Geometry: final body of the model. Coordinates: model frame, mm. A direction names the side the tool comes from. Round coordinates to 2 decimals unless told otherwise and drop trailing zeros. Write each loop counter-clockwise with the first axis right and the second up, starting at its lowest first coordinate (ties: lowest second). Pieces come first, ordered by that corner, then holes. Notation, with made-up numbers: M 18.25,-30.5 L 39.25,-30.5 A14 ccw 39.25,-18.5 Z; hole C 25,13 d4. An arc over 180 degrees is marked long. Use one line per item in the form item = value. Start each with the question number.
Item 1: Reachability of faces 3 (the flat face through (14.53, -6.6, 7.2)), 4 (the flat face through (-5.4, -7.08, -0.9)), 5 (the flat face through (7.4, -7.08, 7.1)), 6 (the flat face through (7, -5.31, 3)), 7 (the flat face through (-3.32, -6.6, -0.9)) from +Z, -Z, +X, -X, +Y, -Y: full face, straight path, thin tool, end or side. Return the list, or none.
Item 2: Pin query (flat end, axial travel): pin 1 Ø5 at (x, z) = (14.5, 3.5) entering from +Y; pin 2 Ø1.1 at (x, z) = (4.5, 7.5) entering from -Y; pin 3 Ø1 at (x, y) = (-2.5, -3.5) entering from -Z; pin 4 Ø0.8 at (x, z) = (15, -1.5) entering from +Y. Return the tip coordinate at first contact, or that it passes through.
Item 3: Section query C-C (x = -8.5). Return loops of the section in (y, z).
Item 4: Pull-direction query (Z, two-part tool) for faces 1 (the flat face through (-21, -1.83, 3)), 2 (the flat face through (1.78, -6.6, -0.9)); classes: pulls with the +Z half, pulls with the -Z half, needs draft (parallel to the pull), parting line crosses it, or undercut.
Item 5: Section query B-B (z = 2.5). State how many separate pieces and enclosed holes the cut face has, and give its area (3 significant figures).
Item 6: Ray query, probe 1 along Z at (x, y) = (-20.5, -5); probe 2 along Z at (x, y) = (-13.5, -1); probe 3 along Y at (x, z) = (7.5, 2.25). Return the intervals inside material, ascending.
Item 7: Section query A-A (y = -2.75). Return loops of the section in (x, z).
from build123d import *

# Parameters (mm, degrees)
SKETCH1_W             = 48.2
SKETCH1_H             = 15.7
MAIN_DEPTH            = 1.6
SKETCH2_W             = 2.54
SKETCH2_H             = 2.54
PINBASE_DEPTH         = 2.54
FILLET1_R             = 0.2
SKETCH3_W             = 1
SKETCH3_H             = 1
BOSS_EXTRUDE3_DEPTH   = 6
LPATTERN3_START       = 1.6
LPATTERN3_DEPTH       = 2.54
LPATTERN3_START_2     = -1.86
LPATTERN3_2_OUTLINE_W = 1
LPATTERN3_2_OUTLINE_H = 1
LPATTERN3_2_DEPTH     = 12
SKETCH5_W             = 8.5
SKETCH5_H             = 10.5
BOSS_EXTRUDE4_DEPTH   = 2.54
SKETCH6_W             = 1.8
SKETCH6_H             = 1.8
CUT_EXTRUDE1_DEPTH    = 6


# Read off the part's stored shape, not the designer's step: LPattern3
with BuildPart() as part:
    # Sketch1 → Main (new body)
    with BuildSketch(Plane.XY):
        Rectangle(SKETCH1_W, SKETCH1_H)
    extrude(amount=MAIN_DEPTH)

    # Sketch2 → PinBase (add)
    with BuildSketch(Plane.XY.offset(1.6)):
        with Locations((15.03, -6.58)):
            Rectangle(SKETCH2_W, SKETCH2_H)
    extrude(amount=PINBASE_DEPTH)

    # Fillet1
    fillet1_edges = [part.edges().sort_by_distance(p)[0] for p in [
        (13.76, -7.85, 2.87),
        (16.3, -7.85, 2.87),
        (16.3, -5.31, 2.87),
    ]]
    fillet(fillet1_edges, radius=FILLET1_R)

    # Sketch3 → Boss-Extrude3 (add, symmetric)
    with BuildSketch(Plane.XY.offset(4.14)):
        with Locations((15.03, -6.58)):
            Rectangle(SKETCH3_W, SKETCH3_H)
    extrude(amount=BOSS_EXTRUDE3_DEPTH, both=True)

    # LPattern3 outline → LPattern3 (add)
    with BuildSketch(Plane.XY.offset(LPATTERN3_START)):
        with BuildLine():
            Line((-6.44, -7.85), (-4.3, -7.85))
            ThreePointArc((-4.3, -7.85), (-4.158578644, -7.791421356), (-4.1, -7.65))
            Line((-4.1, -7.65), (-4.1, -5.51))
            ThreePointArc((-4.1, -5.51), (-4.158578644, -5.368578644), (-4.3, -5.31))
            Line((-4.3, -5.31), (-6.64, -5.31))
            Line((-6.64, -5.31), (-6.64, -7.65))
            ThreePointArc((-6.64, -7.65), (-6.581421356, -7.791421356), (-6.44, -7.85))
        make_face()
        with BuildLine():
            Line((-3.89, -7.85), (-1.75, -7.85))
            ThreePointArc((-1.75, -7.85), (-1.608578644, -7.791421356), (-1.55, -7.65))
            Line((-1.55, -7.65), (-1.55, -5.51))
            ThreePointArc((-1.55, -5.51), (-1.608578644, -5.368578644), (-1.75, -5.31))
            Line((-1.75, -5.31), (-4.09, -5.31))
            Line((-4.09, -5.31), (-4.09, -7.65))
            ThreePointArc((-4.09, -7.65), (-4.031421356, -7.791421356), (-3.89, -7.85))
        make_face()
        with BuildLine():
            Line((-1.34, -7.85), (0.8, -7.85))
            ThreePointArc((0.8, -7.85), (0.941421356, -7.791421356), (1, -7.65))
            Line((1, -7.65), (1, -5.51))
            ThreePointArc((1, -5.51), (0.941421356, -5.368578644), (0.8, -5.31))
            Line((0.8, -5.31), (-1.54, -5.31))
            Line((-1.54, -5.31), (-1.54, -7.65))
            ThreePointArc((-1.54, -7.65), (-1.481421356, -7.791421356), (-1.34, -7.85))
        make_face()
        with BuildLine():
            Line((1.21, -7.85), (3.35, -7.85))
            ThreePointArc((3.35, -7.85), (3.491421356, -7.791421356), (3.55, -7.65))
            Line((3.55, -7.65), (3.55, -5.51))
            ThreePointArc((3.55, -5.51), (3.491421356, -5.368578644), (3.35, -5.31))
            Line((3.35, -5.31), (1.01, -5.31))
            Line((1.01, -5.31), (1.01, -7.65))
            ThreePointArc((1.01, -7.65), (1.068578644, -7.791421356), (1.21, -7.85))
        make_face()
        with BuildLine():
            Line((3.76, -7.85), (5.9, -7.85))
            ThreePointArc((5.9, -7.85), (6.041421356, -7.791421356), (6.1, -7.65))
            Line((6.1, -7.65), (6.1, -5.51))
            ThreePointArc((6.1, -5.51), (6.041421356, -5.368578644), (5.9, -5.31))
            Line((5.9, -5.31), (3.56, -5.31))
            Line((3.56, -5.31), (3.56, -7.65))
            ThreePointArc((3.56, -7.65), (3.618578644, -7.791421356), (3.76, -7.85))
        make_face()
        with BuildLine():
            Line((6.31, -7.85), (8.45, -7.85))
            ThreePointArc((8.45, -7.85), (8.591421356, -7.791421356), (8.65, -7.65))
            Line((8.65, -7.65), (8.65, -5.51))
            ThreePointArc((8.65, -5.51), (8.591421356, -5.368578644), (8.45, -5.31))
            Line((8.45, -5.31), (6.11, -5.31))
            Line((6.11, -5.31), (6.11, -7.65))
            ThreePointArc((6.11, -7.65), (6.168578644, -7.791421356), (6.31, -7.85))
        make_face()
        with BuildLine():
            Line((8.86, -7.85), (11, -7.85))
            ThreePointArc((11, -7.85), (11.141421356, -7.791421356), (11.2, -7.65))
            Line((11.2, -7.65), (11.2, -5.51))
            ThreePointArc((11.2, -5.51), (11.141421356, -5.368578644), (11, -5.31))
            Line((11, -5.31), (8.66, -5.31))
            Line((8.66, -5.31), (8.66, -7.65))
            ThreePointArc((8.66, -7.65), (8.718578644, -7.791421356), (8.86, -7.85))
        make_face()
        with BuildLine():
            Line((11.41, -7.85), (13.55, -7.85))
            ThreePointArc((13.55, -7.85), (13.691421356, -7.791421356), (13.75, -7.65))
            Line((13.75, -7.65), (13.75, -5.51))
            ThreePointArc((13.75, -5.51), (13.691421356, -5.368578644), (13.55, -5.31))
            Line((13.55, -5.31), (11.21, -5.31))
            Line((11.21, -5.31), (11.21, -7.65))
            ThreePointArc((11.21, -7.65), (11.268578644, -7.791421356), (11.41, -7.85))
        make_face()
    extrude(amount=LPATTERN3_DEPTH)

    # LPattern3 2 outline → LPattern3 2 (add)
    with BuildSketch(Plane.XY.offset(LPATTERN3_START_2)):
        with Locations((12.48, -6.58)):
            Rectangle(LPATTERN3_2_OUTLINE_W, LPATTERN3_2_OUTLINE_H)
        with Locations((9.93, -6.58)):
            Rectangle(LPATTERN3_2_OUTLINE_W, LPATTERN3_2_OUTLINE_H)
        with Locations((7.38, -6.58)):
            Rectangle(LPATTERN3_2_OUTLINE_W, LPATTERN3_2_OUTLINE_H)
        with Locations((4.83, -6.58)):
            Rectangle(LPATTERN3_2_OUTLINE_W, LPATTERN3_2_OUTLINE_H)
        with Locations((2.28, -6.58)):
            Rectangle(LPATTERN3_2_OUTLINE_W, LPATTERN3_2_OUTLINE_H)
        with Locations((-0.27, -6.58)):
            Rectangle(LPATTERN3_2_OUTLINE_W, LPATTERN3_2_OUTLINE_H)
        with Locations((-2.82, -6.58)):
            Rectangle(LPATTERN3_2_OUTLINE_W, LPATTERN3_2_OUTLINE_H)
        with Locations((-5.37, -6.58)):
            Rectangle(LPATTERN3_2_OUTLINE_W, LPATTERN3_2_OUTLINE_H)
    extrude(amount=LPATTERN3_2_DEPTH)

    # Sketch5 → Boss-Extrude4 (add)
    with BuildSketch(Plane(origin=(-48.2, 0, 1.6), x_dir=(-1, 0, 0), z_dir=(0, 0, -1))):
        with Locations((-28.35, 0.06)):
            Rectangle(SKETCH5_W, SKETCH5_H)
    extrude(amount=-BOSS_EXTRUDE4_DEPTH)

    # Sketch6 → Cut-Extrude1 (cut)
    with BuildSketch(Plane.ZY.offset(24.1)):
        with Locations((2.87, 3.41)):
            Rectangle(SKETCH6_W, SKETCH6_H)
        with Locations((2.87, 1.24)):
            Rectangle(SKETCH6_W, SKETCH6_H)
        with Locations((2.87, -0.93)):
            Rectangle(SKETCH6_W, SKETCH6_H)
        with Locations((2.87, -3.1)):
            Rectangle(SKETCH6_W, SKETCH6_H)
    extrude(amount=-CUT_EXTRUDE1_DEPTH, mode=Mode.SUBTRACT)


solid = part.part
Working result:
q1.face_3 = +Z, +Y, -Y
q1.face_4 = -Z, +X, -X, -Y
q1.face_5 = +Z, +X, -X, -Y
q1.face_6 = +Z, +X, -X, +Y
q1.face_7 = -Z, +Y, -Y
q2.pin_1 = 7.85
q2.pin_2 = -7.08
q2.pin_3 = 0
q2.pin_4 = -6.08
q3.outline = M -7.85,0 L 7.85,0 L 7.85,1.6 L -7.85,1.6 Z
q4.face_1 = undercut
q4.face_2 = needs draft
q5.separate_pieces = 10
q5.enclosed_holes = 0
q5.area = 104 mm²
q6.probe_1 = 0 to 4.14
q6.probe_2 = 0 to 1.6
q6.probe_3 = -7.85 to -5.31
q7.outline = M -24.1,0 L 24.1,0 L 24.1,1.6 L -15.6,1.6 L -15.6,4.14 L -24.1,4.14 L -24.1,3.77 L -18.1,3.77 L -18.1,1.97 L -24.1,1.97 Z
